```python
from build123d import *

# Parameters (mm, degrees)
SKETCH1_W           = 114.3
SKETCH1_H           = 99.06
BOSS_EXTRUDE1_DEPTH = 9.525
SKETCH1_3_W         = 114.3
SKETCH1_3_H         = 9.525
BOSS_EXTRUDE2_DEPTH = 47.625
SKETCH3_W           = 10.16
SKETCH3_H           = 10.16
SKETCH3_R           = 1.7018
BOSS_EXTRUDE3_DEPTH = 30.48
SKETCH5_W           = 55.88
SKETCH5_H           = 7.239
CUT_EXTRUDE1_DEPTH  = 30.48


with BuildPart() as part:
    # Sketch1 → Boss-Extrude1 (new body)
    with BuildSketch(Plane(origin=(0, 0, 0), x_dir=(1, 0, 0), z_dir=(0, 1, 0))):
        Rectangle(SKETCH1_W, SKETCH1_H)
    extrude(amount=BOSS_EXTRUDE1_DEPTH)

    # Sketch1_3 → Boss-Extrude2 (add)
    with BuildSketch(Plane(origin=(0, 0, 0), x_dir=(1, 0, 0), z_dir=(0, 1, 0))):
        Polygon((-57.15, -49.53), (-57.15, 49.53), (-57.15, 59.055), (-66.675, 59.055), (-66.675, -59.055), (-57.15, -59.055), align=None)
        with Locations((0, 54.2925)):
            Rectangle(SKETCH1_3_W, SKETCH1_3_H)
        Polygon((57.15, 59.055), (57.15, 49.53), (57.15, -49.53), (57.15, -59.055), (66.675, -59.055), (66.675, 59.055), align=None)
        with Locations((0, -54.2925)):
            Rectangle(SKETCH1_3_W, SKETCH1_3_H)
    extrude(amount=BOSS_EXTRUDE2_DEPTH)

    # Sketch3 → Boss-Extrude3 (add)
    with BuildSketch(Plane(origin=(0, 9.525, 0), x_dir=(1, 0, 0), z_dir=(0, 1, 0))):
        with Locations((-52.07, 44.45)):
            Rectangle(SKETCH3_W, SKETCH3_H)
        with Locations((-52.07, 44.45)):
            Circle(SKETCH3_R, mode=Mode.SUBTRACT)
        with Locations((52.07, 44.45)):
            Rectangle(SKETCH3_W, SKETCH3_H)
        with Locations((52.07, 44.45)):
            Circle(SKETCH3_R, mode=Mode.SUBTRACT)
        with Locations((52.07, -44.45)):
            Rectangle(SKETCH3_W, SKETCH3_H)
        with Locations((52.07, -44.45)):
            Circle(SKETCH3_R, mode=Mode.SUBTRACT)
        with Locations((-52.07, -44.45)):
            Rectangle(SKETCH3_W, SKETCH3_H)
        with Locations((-52.07, -44.45)):
            Circle(SKETCH3_R, mode=Mode.SUBTRACT)
    extrude(amount=BOSS_EXTRUDE3_DEPTH)

    # Sketch5 → Cut-Extrude1 (cut)
    with BuildSketch(Plane.ZY.offset(66.675)):
        with Locations((0, 25.4)):
            Rectangle(SKETCH5_W, SKETCH5_H)
    extrude(amount=-CUT_EXTRUDE1_DEPTH, mode=Mode.SUBTRACT)


solid = part.part
```
Geometry check sheet. Reference: the model listing, model coordinates, mm. A direction names the side the tool comes from. Coordinates: 2 decimals unless noted, no trailing zeros. Order: outer loops, then holes, each group sorted by start corner. A loop starts at its lowest first (then second) coordinate and runs counter-clockwise, first axis right, second up. Notation, with made-up numbers: (-39, -14.5) - (-19, -14.5) arc R27 cw to (-19, 21.5) - close; hole circle Ø9 at (43.5, 11.5). An arc over 180 degrees is marked (long way). Answer as a JSON object with one key per item and string values. Group by question number.
Item 1: Sectioned sample at C-C, the plane x = 14. Record the cut outline in (y, z) (3 decimals), and give its area (3 significant figures).
Item 2: Tool access check on faces 1 (the face through (-62, 25, -27.94)), 2 (the face through (1, 23, -59.055)), 3 (the face through (-46.99, 25, -44)). Record the directions out of +Z, -Z, +X, -X, +Y, -Y that give a thin tool (end or side, any length) a straight path to the whole face; none if there is none.
Item 3: Scan lines: probe 1 along Z at (x, y) = (52, 16) (3 decimals); probe 2 along X at (y, z) = (21, -44.45) (3 decimals); probe 3 along Z at (x, y) = (-8, 11) (3 decimals). Record each from-to range of solid material in increasing order.
Item 4: Sectioned sample at A-A, the plane y = 20. Record the cut outline in (x, z) (3 decimals), and give its area (3 significant figures).
Item 5: Depth check by flat-ended pin: pin 1 Ø2 at (x, z) = (29, 36) entering from +Y (3 decimals); pin 2 Ø3 at (x, z) = (-50.5, -42.5) entering from +Y (3 decimals). Enter the tip coordinate at first touch or a pass-through.
Item 6: Sectioned sample at D-D, the plane z = 44.45. Record the cut outline in (x, y) (3 decimals).
Item 7: Draft check along Z on faces 4 (the face through (-62, 25, 27.94)), 5 (the face through (-52.44, 24.55, -42.79)), 6 (the face through (-1, 23, 59.055)), 7 (the face through (66.675, 23, 1)). Enter one of: +Z half, -Z half, draft (parallel to the pull), parting line (faces both ways), or undercut.
Resolved:
{
 "1": {"outline": "(0, -59.055) - (47.625, -59.055) - (47.625, -49.53) - (9.525, -49.53) - (9.525, 49.53) - (47.625, 49.53) - (47.625, 59.055) - (0, 59.055) - close", "area": "1,850 mm^2"},
 "2": {"face 1": "-X", "face 2": "-Z, +X, -X, +Y, -Y", "face 3": "+Y"},
 "3": {"probe 1": "-59.055 to -46.15, -42.75 to -39.37, 39.37 to 42.75, 46.15 to 59.055", "probe 2": "-66.675 to -53.772, -50.368 to -46.99, 46.99 to 50.368, 53.772 to 66.675", "probe 3": "-59.055 to -49.53, 49.53 to 59.055"},
 "4": {"outline": "(-66.675, -59.055) - (66.675, -59.055) - (66.675, 59.055) - (-66.675, 59.055) - close; hole (-57.15, -39.37) - (-46.99, -39.37) - (-46.99, -49.53) - (46.99, -49.53) - (46.99, -39.37) - (57.15, -39.37) - (57.15, 39.37) - (46.99, 39.37) - (46.99, 49.53) - (-46.99, 49.53) - (-46.99, 39.37) - (-57.15, 39.37) - close; hole circle Ø3.404 at (-52.07, -44.45); hole circle Ø3.404 at (-52.07, 44.45); hole circle Ø3.404 at (52.07, -44.45); hole circle Ø3.404 at (52.07, 44.45)", "area": "4,800 mm^2"},
 "5": {"pin 1": "y = 9.525", "pin 2": "y = 40.005"},
 "6": {"outline": "(-66.675, 0) - (66.675, 0) - (66.675, 47.625) - (57.15, 47.625) - (57.15, 40.005) - (53.772, 40.005) - (53.772, 9.525) - (50.368, 9.525) - (50.368, 40.005) - (46.99, 40.005) - (46.99, 9.525) - (-46.99, 9.525) - (-46.99, 40.005) - (-50.368, 40.005) - (-50.368, 9.525) - (-53.772, 9.525) - (-53.772, 40.005) - (-57.15, 40.005) - (-57.15, 47.625) - (-66.675, 47.625) - close"},
 "7": {"face 4": "undercut", "face 5": "undercut", "face 6": "+Z half", "face 7": "draft"}
}
